from build123d import *

# Parameters (mm, degrees)
SKETCH1_R           = 1.5
BOSS_EXTRUDE1_DEPTH = 30
SKETCH2_R           = 2.6
BOSS_EXTRUDE2_DEPTH = 1.7
BOSS_EXTRUDE2_TAPER = 32
SKETCH3_W           = 0.5
SKETCH3_H           = 1.758378485
SKETCH3_H_2         = 1.741621515
SKETCH3_W_2         = 1.734727157
SKETCH3_H_3         = 0.5
SKETCH3_W_3         = 1.765272843
CUT_EXTRUDE1_DEPTH  = 0.3


with BuildPart() as part:
    # Sketch1 → Boss-Extrude1 (new body)
    with BuildSketch(Plane(origin=(0, 0, 0), x_dir=(1, 0, 0), z_dir=(0, 1, 0))):
        Circle(SKETCH1_R)
    extrude(amount=BOSS_EXTRUDE1_DEPTH)

    # Sketch2 → Boss-Extrude2 (add)
    with BuildSketch(Plane(origin=(0, 30, 0), x_dir=(1, 0, 0), z_dir=(0, 1, 0))):
        Circle(SKETCH2_R)
    extrude(amount=-BOSS_EXTRUDE2_DEPTH, taper=BOSS_EXTRUDE2_TAPER)

    # Sketch3 → Cut-Extrude1 (cut)
    with BuildSketch(Plane(origin=(0, 30, 0), x_dir=(1, 0, 0), z_dir=(0, 1, 0))):
        with Locations((-0.015272843, 1.120810757)):
            Rectangle(SKETCH3_W, SKETCH3_H)
        with Locations((-0.015272843, -1.129189243)):
            Rectangle(SKETCH3_W, SKETCH3_H_2)
        with Locations((-1.132636421, -0.008378485)):
            Rectangle(SKETCH3_W_2, SKETCH3_H_3)
        with Locations((1.117363579, -0.008378485)):
            Rectangle(SKETCH3_W_3, SKETCH3_H_3)
        with Locations((-0.015272843, -0.008378485)):
            Rectangle(SKETCH3_W, SKETCH3_H_3)
    extrude(amount=-CUT_EXTRUDE1_DEPTH, mode=Mode.SUBTRACT)


solid = part.part
Could you check a few things on this model? Use its own coordinates, in mm. Round coordinates to 2 decimals unless told otherwise and drop trailing zeros. Write each loop counter-clockwise with the first axis right and the second up, starting at its lowest first coordinate (ties: lowest second). Pieces come first, ordered by that corner, then holes. Notation, with made-up numbers: (16.5, 36.25) - (53.5, 36.25) arc R26 ccw to (53.5, 74.25) - close; hole circle Ø11 at (1.25, 67.5). An arc over 180 degrees is marked (long way). Put each result on its own line as item: value. Start each with the question number.
(1) Will these pins go through, and if not, where does the flat tip stop? pin 1 (3 mm diameter, centred on y = 21, z = -2, fed in from -X); pin 2 (1 mm diameter, centred on x = -0.5, y = 14, fed in from -Z); pin 3 (2 mm diameter, centred on y = 5.5, z = 1.5, fed in from +X); pin 4 (1.2 mm diameter, centred on x = 0, z = 1, fed in from +Y).
(2) Thinking about a two-plate mould opening in X: for faces 1 (the cylindrical face through (-1.5, 13.95, -0.07)), 2 (the flat face through (0, 29.7, 0)), 3 (the flat face through (0, 0, 0)), which applies, released by +X, released by -X, zero draft, split by the parting line, or undercut?
(3) I need wall thicknesses on probe 1 along Y at (x, z) = (-0.2, 1); probe 2 along X at (y, z) = (19, -0.45); probe 3 along X at (y, z) = (4.5, 1.3). Which ranges of each line are inside material? Lowest first, please.
(4) I want a section at A-A, the plane y = 28. Please give me the cut outline in (x, z), plus the area to 3 significant figures.
Here are the results:
1. pin 1: stops at x = -1.41
1. pin 2: stops at z = -1.5
1. pin 3: stops at x = 1.41
1. pin 4: stops at y = 30
2. face 1: split by the parting line
2. face 2: undercut
2. face 3: zero draft
3. probe 1: y = 0 to 29.7
3. probe 2: x = -1.43 to 1.43
3. probe 3: x = -0.75 to 0.75
4. outline: circle Ø3 at (0, 0)
4. area: 7.07 mm^2
